Check sheet for the modelled part. Datum: model origin and axes. Units: mm. Give positions to 0.01 mm unless a question says otherwise; leave off trailing zeros. Order: outer loops, then holes, each group sorted by start corner. A loop starts at its lowest first (then second) coordinate and runs counter-clockwise, first axis right, second up.
```python
from build123d import *

# Parameters (mm, degrees)
F0_W     = 64.466022
F0_H     = 57.840139
F2_DEPTH = 109.263172
F4_DEPTH = 25.4
F6_DEPTH = 80.09805


with BuildPart() as f2:
    # F0 (on Top) → F2 (new body)
    with BuildSketch(Plane.XY):
        with Locations((-16.400989, 28.92007)):
            Rectangle(F0_W, F0_H)
    extrude(amount=F2_DEPTH)

    # F3 (on face) → F4 (cut)
    with BuildSketch(Plane.XZ):
        with BuildLine():
            ThreePointArc((15.832022, 35.303479), (18.376977, 40.519505), (19.251797, 46.256961))
            ThreePointArc((19.251797, 46.256961), (18.376977, 51.994417), (15.832022, 57.210442))
            Line((15.832022, 57.210442), (15.832022, 35.303479))
        make_face()
    extrude(amount=-F4_DEPTH, mode=Mode.SUBTRACT)

    # F5 (on face) → F6 (cut)
    with BuildSketch(Plane.XZ):
        with BuildLine():
            ThreePointArc((15.832022, 57.210442), (-19.251797, 46.256961), (15.832022, 35.303479))
            Line((15.832022, 35.303479), (15.832022, 57.210442))
        make_face()
    extrude(amount=-F6_DEPTH, mode=Mode.SUBTRACT)


solid = f2.part
```
(1) Release check for a two-part mould opening along Z. For faces 1 (the face through (-19.24, 28.52, 46.94)), 2 (the face through (15.832, 29, 17)), 3 (the face through (-17, 29, 0)) record: released by +Z, released by -Z, zero draft, split by the parting line, or undercut.
Response values:
face 1: undercut
face 2: zero draft
face 3: released by -Z
(2) Cross-section at C-C on z = 43. Enter the section's corners in (x, y), then the cut area to 3 significant figures.
Response values:
outline: (-48.63, 0) - (-18.97, 0) - (-18.97, 57.84) - (-48.63, 57.84) - close
area: 1,720 mm2
(3) Gauge pin test, flat end, axial feed: pin 1 Ø23 at (x, z) = (0, 46.26) entering from -Y. Record the tip position at first contact, or that the pin passes through.
Response values:
pin 1: passes through
(4) Cross-section at A-A on x = 0. Enter the section's corners in (y, z), then the cut area to 3 significant figures.
Response values:
outline: (0, 0) - (57.84, 0) - (57.84, 27.01) - (0, 27.01) - close; (0, 65.51) - (57.84, 65.51) - (57.84, 109.26) - (0, 109.26) - close
area: 4,090 mm2
(5) Cross-section at D-D on x = 10. Enter the section's corners in (y, z).
Response values:
outline: (0, 0) - (57.84, 0) - (57.84, 29.81) - (0, 29.81) - close; (0, 62.71) - (57.84, 62.71) - (57.84, 109.26) - (0, 109.26) - close
(6) Cross-section at B-B on y = 52. Enter the section's corners in (x, z).
Response values:
outline: (-48.63, 0) - (15.83, 0) - (15.83, 35.3) arc R19.25 cw (long way) to (15.83, 57.21) - (15.83, 109.26) - (-48.63, 109.26) - close
(7) Material ranges on L1, parallel to Z at x = 0, y = 17; L2, parallel to Z at x = 6.5, y = 24; L3, parallel to X at y = 39, z = 53, recorded low to high.
Response values:
L1: z = 0 to 27.01, 65.51 to 109.26
L2: z = 0 to 28.14, 64.38 to 109.26
L3: x = -48.63 to -18.03
